The listing builds one solid part. Answer for the finished solid, in the listing's coordinates (mm). A direction names the side the tool comes from. Round coordinates to 2 decimals unless told otherwise and drop trailing zeros. Loops run counter-clockwise (first coordinate to the right, second up) from the corner with the lowest first, then second, coordinate; pieces in that order, holes last. Notation, with made-up numbers: M 31,-7.75 L 39,-7.75 A35 ccw 39,29.25 Z; hole C 21.25,-37.75 d11. An arc over 180 degrees is marked long. Put each result on its own line as item: value. Start each with the question number.
(1) Straight lines are drawn through the part: line 1 (Z direction, x = 5, y = 5); line 2 (X direction, y = 30, z = 6.5) (3 decimals); line 3 (Y direction, x = 31, z = 5.08). For each, find the intervals that lie inside material, in ascending order.
(2) Which of the six approach directions +Z, -Z, +X, -X, +Y, -Y give full straight-line access (tool end or side, diameter ignored) to faces 5 (the face through (9.525, 37, 5)), 6 (the face through (25.654, 7, 3)), 7 (the face through (6, 0, 5))?
(3) Section B-B, the plane y = 44.5 is taken. Determine the outline of the cut face in (x, z) (3 decimals), then the cut area to 3 significant figures.
(4) Section D-D, the plane z = 8.75 is taken. Determine the outline of the cut face in (x, y) (3 decimals).
(5) A flat-ended cylindrical pin translates along its axis: P1, Ø5, axis at x = 16.5, z = 6, coming from the -Y side. Find the tip coordinate at first contact, or state that the pin passes through.
(6) Section A-A, the plane z = 5.08 is taken. Determine the outline of the cut face in (x, y) (3 decimals).
(7) Section C-C, the plane x = 26.5 is taken. Determine the outline of the cut face in (y, z).
(8) Determine the mould class of faces 1 (the face through (6, 32, 0)), 2 (the face through (31.79, 3.534, 3.064)), 3 (the face through (6.136, 3.534, 3.064)), 4 (the face through (38.1, 31, 5)) for opening direction Z: released by +Z, released by -Z, zero draft, split by the parting line, or undercut.
```python
from build123d import *

# Parameters (mm, degrees)
BOSS_EXTRUDE2_DEPTH = 10.16
SKETCH4_R           = 2.54
CUT_EXTRUDE1_DEPTH  = 38.1


with BuildPart() as part:
    # Sketch1 → Boss-Extrude2 (new body)
    with BuildSketch(Plane.XY):
        Polygon((0, 0), (12.446, 0), (12.446, 10.16), (25.654, 10.16), (25.654, 0), (38.1, 0), (38.1, 63.5), (0, 63.5), align=None)
        with BuildLine():
            Line((9.525, 49.078456098), (9.525, 23.678456098))
            ThreePointArc((9.525, 23.678456098), (19.05, 14.153456098), (28.575, 23.678456098))
            Line((28.575, 23.678456098), (28.575, 49.078456098))
            ThreePointArc((28.575, 49.078456098), (19.05, 58.603456098), (9.525, 49.078456098))
        make_face(mode=Mode.SUBTRACT)
    extrude(amount=BOSS_EXTRUDE2_DEPTH)

    # Sketch4 → Cut-Extrude1 (cut)
    with BuildSketch(Plane.ZY):
        with Locations((5.08, 5.08)):
            Circle(SKETCH4_R)
    extrude(amount=-CUT_EXTRUDE1_DEPTH, mode=Mode.SUBTRACT)


solid = part.part
```
Recorded:
1. line 1: z = 0 to 2.54, 7.62 to 10.16
1. line 2: x = 0 to 9.525, 28.575 to 38.1
1. line 3: y = 0 to 2.54, 7.62 to 63.5
2. face 5: +Z, -Z
2. face 6: +Z, -Z, -Y
2. face 7: +Z, -Z, +X, -X, -Y
3. outline: M 0,0 L 9.525,0 L 9.525,10.16 L 0,10.16 Z; M 28.575,0 L 38.1,0 L 38.1,10.16 L 28.575,10.16 Z
3. area: 194 mm²
4. outline: M 0,0 L 12.446,0 L 12.446,10.16 L 25.654,10.16 L 25.654,0 L 38.1,0 L 38.1,63.5 L 0,63.5 Z; hole M 9.525,23.678 A9.525 ccw 28.575,23.678 L 28.575,49.078 A9.525 ccw 9.525,49.078 Z
5. P1: stops at y = 10.16
6. outline: M 0,0 L 12.446,0 L 12.446,2.54 L 0,2.54 Z; M 0,7.62 L 12.446,7.62 L 12.446,10.16 L 25.654,10.16 L 25.654,7.62 L 38.1,7.62 L 38.1,63.5 L 0,63.5 Z; M 25.654,0 L 38.1,0 L 38.1,2.54 L 25.654,2.54 Z; hole M 9.525,23.678 A9.525 ccw 28.575,23.678 L 28.575,49.078 A9.525 ccw 9.525,49.078 Z
7. outline: M 0,0 L 17.74,0 L 17.74,10.16 L 0,10.16 Z; M 55.01,0 L 63.5,0 L 63.5,10.16 L 55.01,10.16 Z; hole C 5.08,5.08 d5.08
8. face 1: released by -Z
8. face 2: undercut
8. face 3: undercut
8. face 4: zero draft
